```python
from build123d import *

# Parameters (mm, degrees)
SKETCH2_W               = 609.6
SKETCH2_H               = 3.175
CHAMFER1_SIZE           = 0.9525
CUT_EXTRUDE1_DEPTH      = 305.833071123
CUT_EXTRUDE1_DEPTH_BACK = 305.833071123
SKETCH5_W               = 254
SKETCH5_H               = 50.8


with BuildPart() as part:
    # Sketch2 → Revolve1 (revolve)
    with BuildSketch(Plane(origin=(0, 0, 0), x_dir=(0, 0, -1), z_dir=(1, 0, 0)), mode=Mode.PRIVATE) as revolve1_sk:
        with Locations((0, 1.5875)):
            Rectangle(SKETCH2_W, SKETCH2_H)
    revolve(revolve1_sk.sketch.rotate(Axis((0, 0, 304.8), (0, 0, -1)), 90), axis=Axis((0, 0, 304.8), (0, 0, -1)))

    # Chamfer1
    chamfer1_edges = [part.edges().sort_by_distance(p)[0] for p in [
        (-3.175, 0, -304.8),
        (-3.175, 0, 304.8),
    ]]
    chamfer(chamfer1_edges, length=CHAMFER1_SIZE)

    # Sketch5 → Cut-Extrude1 (cut, two sides: drawn at the far end of the back side and taken through both)
    with BuildSketch(Plane(origin=(0, 0, 0), x_dir=(0, 0, -1), z_dir=(1, 0, 0)).offset(-CUT_EXTRUDE1_DEPTH_BACK)):
        with Locations((177.8, 0)):
            Rectangle(SKETCH5_W, SKETCH5_H)
    extrude(amount=CUT_EXTRUDE1_DEPTH + CUT_EXTRUDE1_DEPTH_BACK, mode=Mode.SUBTRACT)


solid = part.part
```
Can you work these out from the model? Positions are in its coordinate system, mm. Coordinates: 2 decimals unless noted, no trailing zeros. Loops run counter-clockwise (first coordinate to the right, second up) from the corner with the lowest first, then second, coordinate; pieces in that order, holes last. Notation, with made-up numbers: (55, -39) -> (96, -39) arc R22 ccw to (96, -3) -> close; hole circle Ø5 at (-28.75, 32.25). An arc over 180 degrees is marked (long way). Put each result on its own line as item: value. Start each with the question number.
Q1. I'm going to push a flat-ended pin straight in: P1, Ø2, axis at x = 2.5, y = 2, coming from the -Z side. Where does the tip first touch, or does it pass through?
Q2. I want a section at A-A (z = 104). Write out the boundary of the cut face in (x, y) (3 decimals).
Q3. If I drill on line 1 (Y direction, x = 0.25, z = 7.5); line 2 (Y direction, x = -0.5, z = 35.5); line 3 (X direction, y = 2.25, z = 240), over which ranges is the centre line in solid material (lowest first)? Write a range as [from, to].
Taken from the geometry:
1. P1: stops at z = -50.8
2. outline: circle Ø6.35 at (0, 0)
3. line 1: y = [-3.17, 3.17]
3. line 2: y = [-3.14, 3.14]
3. line 3: x = [-2.24, 2.24]
